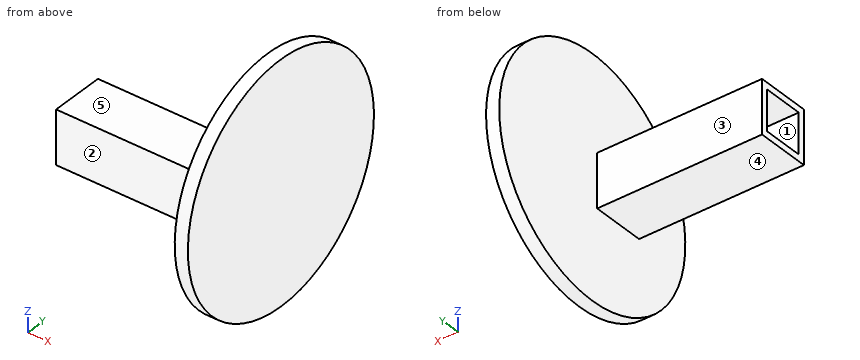
Autodesk Inventor part; units mm, degrees
ref_plane "YZ Plane" through (0, 0, 0) normal (1, 0, 0) x (0, 1, 0)
ref_plane "XZ Plane" through (0, 0, 0) normal (0, 1, 0) x (-1, 0, 0)
ref_plane "XY Plane" through (0, 0, 0) normal (0, 0, 1) x (1, 0, 0)
sketch "Sketch3" plane through (0, 0, 0) normal (1, 0, 0) x (0, 1, 0)
  line L0 (3.05, -3.05) -> (-3.05, -3.05)
  line L1 (-3.05, -3.05) -> (-3.05, 3.05)
  line L2 (-3.05, 3.05) -> (3.05, 3.05)
  line L3 (3.05, 3.05) -> (3.05, -3.05)
  line L4 (3.05, -3.05) -> (-3.05, 3.05) construction
  line L5 (-3.05, -3.05) -> (3.05, 3.05) construction
  line L6 (4.05, -4.05) -> (-4.05, -4.05)
  line L7 (-4.05, -4.05) -> (-4.05, 4.05)
  line L8 (-4.05, 4.05) -> (4.05, 4.05)
  line L9 (4.05, 4.05) -> (4.05, -4.05)
  line L10 (4.05, -4.05) -> (-4.05, 4.05) construction
  line L11 (-4.05, -4.05) -> (4.05, 4.05) construction
  point P0 (0, 0)
  point P1 (0, 0)
  point P2 (0, 0)
  dimension "d38" = 8.1
  dimension "d39" = 8.1
  dimension "d40" = 6.1
  dimension "d41" = 6.1
extrude "Extrusion2" add sketch "Sketch3" along normal blind 25
sketch "Sketch9" plane through (25, 0, 0) normal (1, 0, 0) x (0, 0, -1)
  line L0 (-4.05, 4.05) -> (-4.05, -4.05)
  line L1 (-4.05, -4.05) -> (4.05, -4.05)
  line L2 (4.05, -4.05) -> (4.05, 4.05)
  line L3 (4.05, 4.05) -> (-4.05, 4.05)
  line L4 (3.05, 3.05) -> (3.05, -3.05)
  line L5 (3.05, -3.05) -> (-3.05, -3.05)
  line L6 (-3.05, -3.05) -> (-3.05, 3.05)
  line L7 (-3.05, 3.05) -> (3.05, 3.05)
  circle A0 centre (0, 5) radius 18
  line L8 (0, 0) -> (0, 9.371) construction
  dimension "d42" = 5
  dimension "d45" = 36
extrude "Extrusion6" add sketch "Sketch9" along normal blind 2 contours L3 L2 L1 L0 | L4 L5 L6 L7 | A0
equation "\"d39\" = d38"
properties part number "propellor_fuselage_interface" material "Nylon 6/6"
Could you check a few things on this model? Use its own coordinates, in mm. Face numbers are marked on the shaded views. A direction names the side the tool comes from. Round coordinates to 2 decimals unless told otherwise and drop trailing zeros. Write each loop counter-clockwise with the first axis right and the second up, starting at its lowest first coordinate (ties: lowest second). Pieces come first, ordered by that corner, then holes. Notation, with made-up numbers: (66, 22.5) - (100, 22.5) arc R16 ccw to (100, 43.5) - close; hole circle Ø8 at (1, -9). An arc over 180 degrees is marked (long way). Use a Markdown table: item, result.
Q1. I want a section at B-B (z = 0). List the corners of the cut face in (x, y) for me.
Output values:
| item | result |
|---|---|
| outline | (0, -4.05) - (25, -4.05) - (25, -13) - (27, -13) - (27, 23) - (25, 23) - (25, 4.05) - (0, 4.05) - (0, 3.05) - (25, 3.05) - (25, -3.05) - (0, -3.05) - close |
Q2. For pin 1 (9 mm diameter, centred on x = 10, z = 0, fed in from -Y); pin 2 (2.5 mm diameter, centred on x = 7.5, y = 0.5, fed in from +Z); pin 3 (5 mm diameter, centred on x = 24, z = 13.5, fed in from +Y), each with a flat end and sliding along its axis, tell me the tip position at first contact or that it passes through.
Output values:
| item | result |
|---|---|
| pin 1 | y = -4.05 |
| pin 2 | z = 4.05 |
| pin 3 | y = 19.08 |
Q3. I want a section at D-D (y = 5). List the corners of the cut face in (x, z) for me.
Output values:
| item | result |
|---|---|
| outline | (25, -18) - (27, -18) - (27, 18) - (25, 18) - close |
Q4. I want a section at C-C (y = -2). List the corners of the cut face in (x, z) for me, plus the area to 3 significant figures.
Output values:
| item | result |
|---|---|
| outline | (0, -4.05) - (25, -4.05) - (25, -16.58) - (27, -16.58) - (27, 16.58) - (25, 16.58) - (25, 4.05) - (0, 4.05) - (0, 3.05) - (25, 3.05) - (25, -3.05) - (0, -3.05) - close |
| area | 116 mm2 |
Q5. I want a section at A-A (x = 7.75). List the corners of the cut face in (y, z) for me, plus the area to 3 significant figures.
Output values:
| item | result |
|---|---|
| outline | (-4.05, -4.05) - (4.05, -4.05) - (4.05, 4.05) - (-4.05, 4.05) - close; hole (-3.05, -3.05) - (3.05, -3.05) - (3.05, 3.05) - (-3.05, 3.05) - close |
| area | 28.4 mm2 |
Q6. For the marked faces 1, 2, 3, 4 and 5, which set-ups out of +Z, -Z, +X, -X, +Y, -Y let a thin tool reach every point of the face, with its end or its side?
Output values:
| item | result |
|---|---|
| face 1 | -X |
| face 2 | +Z, -Z, -X, -Y |
| face 3 | +Z, -Z, -X, +Y |
| face 4 | -Z, -X, +Y, -Y |
| face 5 | +Z, -X, +Y, -Y |
Q7. Please list where these lines run through material, in increasing order: L1, parallel to Y at x = 9.5, z = 2; L2, parallel to X at y = -8.5, z = 5.
Output values:
| item | result |
|---|---|
| L1 | -4.05 to -3.05, 3.05 to 4.05 |
| L2 | 25 to 27 |
